Could you check a few things on this model? Use its own coordinates, in mm. Face numbers are marked on the shaded views. A direction names the side the tool comes from. Round coordinates to 2 decimals unless told otherwise and drop trailing zeros. Loops run counter-clockwise (first coordinate to the right, second up) from the corner with the lowest first, then second, coordinate; pieces in that order, holes last. Notation, with made-up numbers: M 44,-10.5 L 78,-10.5 A18 ccw 78,10.5 Z; hole C 89,-1.75 d10. An arc over 180 degrees is marked long. Answer in a Markdown table with one row per item.
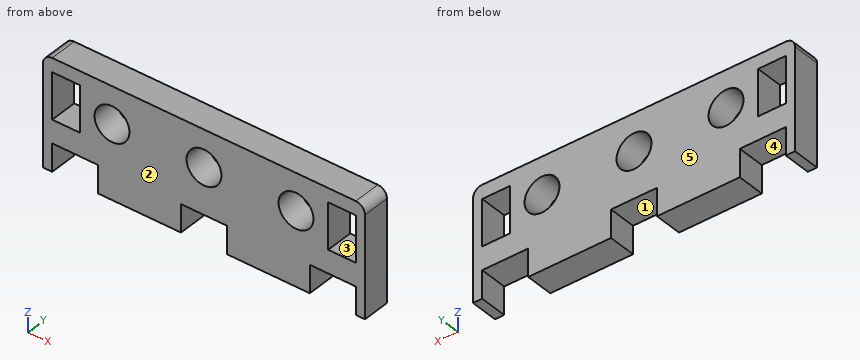
```python
from build123d import *

# Parameters (mm, degrees)
SKETCH1_W             = 35
SKETCH1_H             = 12
BOSS_EXTRUDE1_DEPTH   = 3
SKETCH5_W             = 3
SKETCH5_H             = 5
SKETCH5_W_2           = 5
SKETCH5_H_2           = 3
CUT_EXTRUDE1_DEPTH    = 3
FILLET1_R             = 1
F_6_CLEARANCE_HOLE2_D = 3.7973


with BuildPart() as part:
    # Sketch1 → Boss-Extrude1 (new body)
    with BuildSketch(Plane(origin=(0, 0, 0), x_dir=(1, 0, 0), z_dir=(0, 1, 0))):
        Rectangle(SKETCH1_W, SKETCH1_H)
    extrude(amount=BOSS_EXTRUDE1_DEPTH)

    # Sketch5 → Cut-Extrude1 (cut)
    with BuildSketch(Plane(origin=(0, 3, 0), x_dir=(1, 0, 0), z_dir=(0, 1, 0))):
        with Locations((-15, -2)):
            Rectangle(SKETCH5_W, SKETCH5_H)
        with Locations((15, -2)):
            Rectangle(SKETCH5_W, SKETCH5_H)
        with Locations((-14, 4.5)):
            Rectangle(SKETCH5_W_2, SKETCH5_H_2)
        with Locations((0, 4.5)):
            Rectangle(SKETCH5_W_2, SKETCH5_H_2)
        with Locations((14, 4.5)):
            Rectangle(SKETCH5_W_2, SKETCH5_H_2)
    extrude(amount=-CUT_EXTRUDE1_DEPTH, mode=Mode.SUBTRACT)

    # Fillet1
    fillet1_edges = [part.edges().sort_by_distance(p)[0] for p in [
        (-17.5, 1.5, 6),
        (17.5, 1.5, 6),
    ]]
    fillet(fillet1_edges, radius=FILLET1_R)

    # #6 Clearance Hole2 (through all)
    with Locations(Plane(origin=(0, 3, 0), x_dir=(1, 0, 0), z_dir=(0, 1, 0))):
        with Locations((-10, -2), (0, -2), (10, -2)):
            Hole(F_6_CLEARANCE_HOLE2_D / 2)


solid = part.part
```
1) I want a section at B-B, the plane z = 2. Please give me the cut outline in (x, y).
Computed:
| item | result |
|---|---|
| outline | M -17.5,0 L -16.5,0 L -16.5,3 L -17.5,3 Z; M -13.5,0 L -11.9,0 L -11.9,3 L -13.5,3 Z; M -8.1,0 L -1.9,0 L -1.9,3 L -8.1,3 Z; M 1.9,0 L 8.1,0 L 8.1,3 L 1.9,3 Z; M 11.9,0 L 13.5,0 L 13.5,3 L 11.9,3 Z; M 16.5,0 L 17.5,0 L 17.5,3 L 16.5,3 Z |
2) I want a section at C-C, the plane y = 1.3. State how many separate pieces and enclosed holes the cut face has, plus the area to 3 significant figures.
Computed:
| item | result |
|---|---|
| separate pieces | 1 |
| enclosed holes | 5 |
| area | 311 mm² |
3) I want a section at A-A, the plane x = 14. Please give me the cut outline in (y, z), plus the area to 3 significant figures.
Computed:
| item | result |
|---|---|
| outline | M 0,-3 L 3,-3 L 3,-0.5 L 0,-0.5 Z; M 0,4.5 L 3,4.5 L 3,6 L 0,6 Z |
| area | 12.0 mm² |
4) I need wall thicknesses on line 1 (X direction, y = 1.7, z = -4); line 2 (Z direction, x = 10, y = 0.8); line 3 (X direction, y = 1.15, z = 3.25). Which ranges of each line are inside material? Lowest first, please.
Computed:
| item | result |
|---|---|
| line 1 | x = -17.5 to -16.5, -11.5 to -2.5, 2.5 to 11.5, 16.5 to 17.5 |
| line 2 | z = -6 to 0.1, 3.9 to 6 |
| line 3 | x = -17.5 to -16.5, -13.5 to -11.43, -8.57 to -1.43, 1.43 to 8.57, 11.43 to 13.5, 16.5 to 17.5 |
5) If we mould it in two halves opening along X, with no side actions, what happens to the marked faces 4 and 5? For each: released by +X, released by -X, zero draft, split by the parting line, or undercut.
Computed:
| item | result |
|---|---|
| face 4 | undercut |
| face 5 | zero draft |
6) Will this pin go through, and if not, where does the flat tip stop? P1, Ø1.5, axis at x = -15.5, y = 2, coming from the -Z side.
Computed:
| item | result |
|---|---|
| P1 | stops at z = -3 |
7) I want a section at D-D, the plane x = 10. Please give me the cut outline in (y, z).
Computed:
| item | result |
|---|---|
| outline | M 0,-6 L 3,-6 L 3,0.1 L 0,0.1 Z; M 0,3.9 L 3,3.9 L 3,6 L 0,6 Z |
8) Which directions (+Z, -Z, +X, -X, +Y, -Y) give clear straight access to the entire face, cutting with the end or side of a thin tool? Please do the marked faces 1, 2 and 3.
Computed:
| item | result |
|---|---|
| face 1 | -Z, +Y, -Y |
| face 2 | +Z, -Z, +X, -X, -Y |
| face 3 | +Y, -Y |
